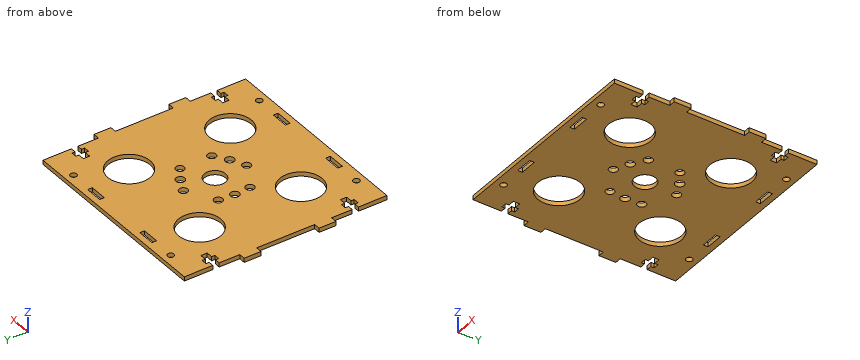
from build123d import *

# Parameters (mm, degrees)
SKETCH_1_R      = 1.5
SKETCH_1_R_2    = 2
SKETCH_1_R_3    = 2.08
SKETCH_1_R_4    = 5
SKETCH_1_R_5    = 10
SKETCH_1_W      = 8.2
SKETCH_1_H      = 2.2
EXTRUDE_1_DEPTH = 2


with BuildPart() as part:
    # 草图1 → 凸台-拉伸1 (new body)
    with BuildSketch(Plane.XY):
        Polygon((-50.266155614, -92.324512395), (-50.266155614, -102.074512395), (-47.766155614, -102.074512395), (-47.766155614, -100.574512395), (-45.166155614, -100.574512395), (-45.166155614, -102.074512395), (-42.166155614, -102.074512395), (-42.166155614, -105.074512395), (-45.166155614, -105.074512395), (-45.166155614, -106.574512395), (-47.766155614, -106.574512395), (-47.766155614, -105.074512395), (-50.266155614, -105.074512395), (-50.266155614, -106.074512395), (-50.266155614, -118.574512395), (-2.266155614, -118.574512395), (45.733844386, -118.574512395), (45.733844386, -106.074512395), (45.733844386, -105.074512395), (43.233844386, -105.074512395), (43.233844386, -106.574512395), (40.633844386, -106.574512395), (40.633844386, -105.074512395), (37.633844386, -105.074512395), (37.633844386, -102.074512395), (40.633844386, -102.074512395), (40.633844386, -100.574512395), (43.233844386, -100.574512395), (43.233844386, -102.074512395), (45.733844386, -102.074512395), (45.733844386, -92.324512395), (48.733844386, -92.324512395), (48.733844386, -84.324512395), (45.733844386, -84.324512395), (45.733844386, -56.824512395), (48.733844386, -56.824512395), (48.733844386, -48.824512395), (45.733844386, -48.824512395), (45.733844386, -39.074512395), (43.233844386, -39.074512395), (43.233844386, -40.574512395), (40.633844386, -40.574512395), (40.633844386, -39.074512395), (37.633844386, -39.074512395), (37.633844386, -36.074512395), (40.633844386, -36.074512395), (40.633844386, -34.574512395), (43.233844386, -34.574512395), (43.233844386, -36.074512395), (45.733844386, -36.074512395), (45.733844386, -23.574512395), (45.733844386, -22.574512395), (-2.266155614, -22.574512395), (-50.266155614, -22.574512395), (-50.266155614, -23.574512395), (-50.266155614, -36.074512395), (-47.766155614, -36.074512395), (-47.766155614, -34.574512395), (-45.166155614, -34.574512395), (-45.166155614, -36.074512395), (-42.166155614, -36.074512395), (-42.166155614, -39.074512395), (-45.166155614, -39.074512395), (-45.166155614, -40.574512395), (-47.766155614, -40.574512395), (-47.766155614, -39.074512395), (-50.266155614, -39.074512395), (-50.266155614, -48.824512395), (-53.266155614, -48.824512395), (-53.266155614, -56.824512395), (-50.266155614, -56.824512395), (-50.266155614, -84.324512395), (-53.266155614, -84.324512395), (-53.266155614, -92.324512395), align=None)
        with Locations((-35.266155614, -114.574512396)):
            Circle(SKETCH_1_R, mode=Mode.SUBTRACT)
        with Locations(Location((30.733844386, -114.574512396, 0), (0, 0, 180))):
            Circle(SKETCH_1_R, mode=Mode.SUBTRACT)
        with Locations((30.733844386, -26.574512395)):
            Circle(SKETCH_1_R, mode=Mode.SUBTRACT)
        with Locations(Location((-35.266155614, -26.574512395, 0), (0, 0, 180))):
            Circle(SKETCH_1_R, mode=Mode.SUBTRACT)
        with Locations((-2.266155614, -85.571739483)):
            Circle(SKETCH_1_R_2, mode=Mode.SUBTRACT)
        with Locations((-15.254135258, -78.073125939)):
            Circle(SKETCH_1_R_2, mode=Mode.SUBTRACT)
        with Locations((-15.254135258, -63.075898852)):
            Circle(SKETCH_1_R_2, mode=Mode.SUBTRACT)
        with Locations((-2.266155614, -55.577285308)):
            Circle(SKETCH_1_R_2, mode=Mode.SUBTRACT)
        with Locations((10.721824031, -63.075898852)):
            Circle(SKETCH_1_R_2, mode=Mode.SUBTRACT)
        with Locations((10.721824031, -78.073125939)):
            Circle(SKETCH_1_R_2, mode=Mode.SUBTRACT)
        with Locations((-15.796155614, -70.574512395)):
            Circle(SKETCH_1_R_3, mode=Mode.SUBTRACT)
        with Locations((4.498844386, -58.857188682)):
            Circle(SKETCH_1_R_3, mode=Mode.SUBTRACT)
        with Locations((4.498844386, -82.291836109)):
            Circle(SKETCH_1_R_3, mode=Mode.SUBTRACT)
        with Locations((-2.266155614, -70.574512395)):
            Circle(SKETCH_1_R_4, mode=Mode.SUBTRACT)
        with Locations((-26.266155614, -46.574512395)):
            Circle(SKETCH_1_R_5, mode=Mode.SUBTRACT)
        with Locations((21.733844386, -46.574512395)):
            Circle(SKETCH_1_R_5, mode=Mode.SUBTRACT)
        with Locations((21.733844386, -94.574512395)):
            Circle(SKETCH_1_R_5, mode=Mode.SUBTRACT)
        with Locations((-26.266155614, -94.574512395)):
            Circle(SKETCH_1_R_5, mode=Mode.SUBTRACT)
        with Locations((-20.016155614, -114.574512396)):
            Rectangle(SKETCH_1_W, SKETCH_1_H, mode=Mode.SUBTRACT)
        with Locations((15.483844386, -114.574512396)):
            Rectangle(SKETCH_1_W, SKETCH_1_H, mode=Mode.SUBTRACT)
        with Locations((15.483844386, -26.574512395)):
            Rectangle(SKETCH_1_W, SKETCH_1_H, mode=Mode.SUBTRACT)
        with Locations((-20.016155614, -26.574512395)):
            Rectangle(SKETCH_1_W, SKETCH_1_H, mode=Mode.SUBTRACT)
    extrude(amount=EXTRUDE_1_DEPTH)


solid = part.part
The listing builds one solid part. Answer for the finished solid, in the listing's coordinates (mm). Coordinates: 2 decimals unless noted, no trailing zeros. Loops run counter-clockwise (first coordinate to the right, second up) from the corner with the lowest first, then second, coordinate; pieces in that order, holes last.
1) Find the intervals of material crossed by L1, parallel to Y at x = -2, z = 0.85; L2, parallel to Y at x = 41.5, z = 1.05; L3, parallel to Y at x = 21.5, z = 0.3, in increasing order.
2) Find section C-C on y = -108.5. Write down the section's boundary in (x, z).
3) Find section A-A on x = 30.5. Write down the section's boundary in (y, z).
4) Find section B-B on y = -44. Write down the section's boundary in (x, z).
5) Find section D-D on z = 1.35. Give the number of separate pieces and of enclosed holes in the cut face, then the cut area to 3 significant figures.
6) Flat-ended cylindrical pins translate along their axes: pin 1 Ø1 at (y, z) = (-114.5, 1) entering from -X; pin 2 Ø1.5 at (x, y) = (-3.5, -73) entering from +Z; pin 3 Ø0.6 at (x, z) = (-52.5, 1) entering from -Y. Find the tip coordinate at first contact, or state that the pin passes through.
Values:
1. L1: y = -118.57 to -87.55, -83.59 to -75.57, -65.58 to -57.56, -53.6 to -22.57
1. L2: y = -118.57 to -106.57, -100.57 to -40.57, -34.57 to -22.57
1. L3: y = -118.57 to -104.57, -84.58 to -56.57, -36.58 to -22.57
2. outline: (-50.27, 0) - (45.73, 0) - (45.73, 2) - (-50.27, 2) - close
3. outline: (-118.57, 0) - (-116.06, 0) - (-116.06, 2) - (-118.57, 2) - close; (-113.09, 0) - (-99.39, 0) - (-99.39, 2) - (-113.09, 2) - close; (-89.76, 0) - (-51.39, 0) - (-51.39, 2) - (-89.76, 2) - close; (-41.76, 0) - (-28.06, 0) - (-28.06, 2) - (-41.76, 2) - close; (-25.09, 0) - (-22.57, 0) - (-22.57, 2) - (-25.09, 2) - close
4. outline: (-50.27, 0) - (-35.93, 0) - (-35.93, 2) - (-50.27, 2) - close; (-16.6, 0) - (12.07, 0) - (12.07, 2) - (-16.6, 2) - close; (31.4, 0) - (45.73, 0) - (45.73, 2) - (31.4, 2) - close
5. separate pieces: 1
5. enclosed holes: 22
5. area: 7,630 mm2
6. pin 1: stops at x = -50.27
6. pin 2: passes through
6. pin 3: stops at y = -92.32
